Source: CAD feature listing. Evaluate the final solid. Frame: model axes, mm. Give positions to 0.01 mm unless a question says otherwise; leave off trailing zeros. Loops run counter-clockwise (first coordinate to the right, second up) from the corner with the lowest first, then second, coordinate; pieces in that order, holes last. Notation, with made-up numbers: M 72,60.5 L 113,60.5 A11 cw 113,68.5 Z; hole C 59,62 d7. An arc over 180 degrees is marked long. Answer in a Markdown table with one row per item.
```python
from build123d import *

# Parameters (mm, degrees)
F1_W     = 75
F1_H     = 75
F2_DEPTH = 0.45
F3_DEPTH = 0.451
F4_SCALE = 2
F5_R     = 10


with BuildPart() as f2:
    # F1 (on Top) → F2 (new body)
    with BuildSketch(Plane.XY):
        with Locations((42.972257086, 25.7581188657)):
            Rectangle(F1_W, F1_H)
    extrude(amount=F2_DEPTH)

    # F0 (on Top) → F3 (cut, through all)
    with BuildSketch(Plane.XY):
        with BuildLine():
            Line((20.8079852164, 34.7860567272), (63.291762352, 34.7860567272))
            ThreePointArc((63.291762352, 34.7860567272), (64.7059759144, 35.3718431648), (65.291762352, 36.7860567272))
            Line((65.291762352, 36.7860567272), (65.291762352, 39.0860567272))
            Line((65.291762352, 39.0860567272), (22.8079852164, 39.0860567272))
            ThreePointArc((22.8079852164, 39.0860567272), (21.393771654, 38.5002702895), (20.8079852164, 37.0860567272))
            Line((20.8079852164, 37.0860567272), (20.8079852164, 34.7860567272))
        make_face()
        with BuildLine():
            Line((38.5079852164, 14.3860567272), (38.5079852164, 32.2860567272))
            Line((38.5079852164, 32.2860567272), (31.5079852164, 32.2860567272))
            ThreePointArc((31.5079852164, 32.2860567272), (30.093771654, 31.7002702895), (29.5079852164, 30.2860567272))
            Line((29.5079852164, 30.2860567272), (29.5079852164, 12.3860567272))
            Line((29.5079852164, 12.3860567272), (36.5079852164, 12.3860567272))
            ThreePointArc((36.5079852164, 12.3860567272), (37.9221987788, 12.9718431648), (38.5079852164, 14.3860567272))
        make_face()
        with BuildLine():
            Line((54.1434029907, 27.9860567272), (54.1434029907, 32.2860567272))
            Line((54.1434029907, 32.2860567272), (47.1434029907, 32.2860567272))
            ThreePointArc((47.1434029907, 32.2860567272), (45.7291894283, 31.7002702895), (45.1434029907, 30.2860567272))
            Line((45.1434029907, 30.2860567272), (45.1434029907, 12.3860567272))
            Line((45.1434029907, 12.3860567272), (54.1434029907, 12.3860567272))
            Line((54.1434029907, 12.3860567272), (54.1434029907, 16.6860567272))
            Line((54.1434029907, 16.6860567272), (54.1434029907, 23.6860567272))
            Line((54.1434029907, 23.6860567272), (54.1434029907, 27.9860567272))
        make_face()
        with BuildLine():
            Line((65.291762352, 27.9860567272), (54.1434029907, 27.9860567272))
            Line((54.1434029907, 27.9860567272), (54.1434029907, 23.6860567272))
            Line((54.1434029907, 23.6860567272), (63.291762352, 23.6860567272))
            ThreePointArc((63.291762352, 23.6860567272), (64.7059759144, 24.2718431648), (65.291762352, 25.6860567272))
            Line((65.291762352, 25.6860567272), (65.291762352, 27.9860567272))
        make_face()
        with BuildLine():
            Line((65.291762352, 16.6860567272), (54.1434029907, 16.6860567272))
            Line((54.1434029907, 16.6860567272), (54.1434029907, 12.3860567272))
            Line((54.1434029907, 12.3860567272), (63.291762352, 12.3860567272))
            ThreePointArc((63.291762352, 12.3860567272), (64.7059759144, 12.9718431648), (65.291762352, 14.3860567272))
            Line((65.291762352, 14.3860567272), (65.291762352, 16.6860567272))
        make_face()
    extrude(amount=F3_DEPTH, mode=Mode.SUBTRACT)


with BuildPart() as f2_1:
    # F4: moved
    add(f2.part.scale(F4_SCALE))

    # F5
    f5_edges = [f2_1.edges().sort_by_distance(p)[0] for p in [
        (160.944514, -23.483762, 0.45),
        (10.944514, -23.483762, 0.45),
        (10.944514, 126.516238, 0.45),
        (160.944514, 126.516238, 0.45),
    ]]
    fillet(f5_edges, radius=F5_R)


solid = f2_1.part
```
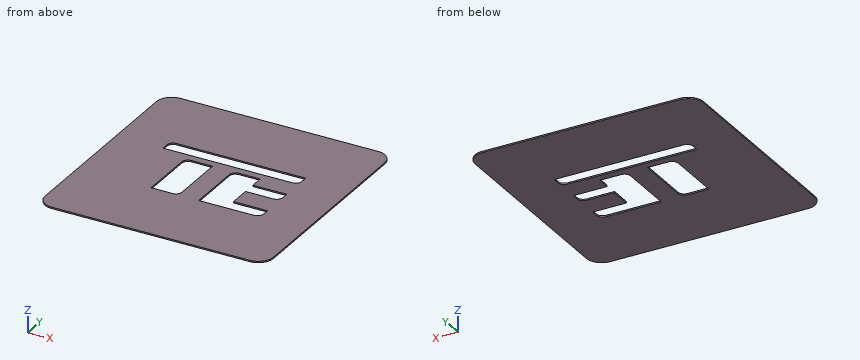
Q1. Section query C-C (y = 42.5). Output: boundary loops of the cut face in (x, z), plus the area to 3 significant figures.
Values follow:
| item | result |
|---|---|
| outline | M 10.94,0 L 59.02,0 L 59.02,0.9 L 10.94,0.9 Z; M 77.02,0 L 90.29,0 L 90.29,0.9 L 77.02,0.9 Z; M 108.29,0 L 160.94,0 L 160.94,0.9 L 108.29,0.9 Z |
| area | 103 mm^2 |
Q2. Section query B-B (z = 0.3). Give the number of separate pieces and of enclosed holes in the cut face, plus the area to 3 significant figures.
Values follow:
| item | result |
|---|---|
| separate pieces | 1 |
| enclosed holes | 3 |
| area | 19,900 mm^2 |
Q3. Ray query, probe 1 along X at (y, z) = (61, 0.65); probe 2 along Y at (x, z) = (118, 0.55); probe 3 along Y at (x, z) = (69.5, 0.8). Return the intervals inside material, ascending. Write a range as from..to.
Values follow:
| item | result |
|---|---|
| probe 1 | 10.94..59.04, 77.02..90.31, 108.29..160.94 |
| probe 2 | -23.48..24.77, 33.37..47.37, 55.97..69.57, 78.17..126.52 |
| probe 3 | -23.48..24.77, 64.57..69.57, 78.17..126.52 |
Q4. Section query A-A (x = 96). Output: boundary loops of the cut face in (y, z).
Values follow:
| item | result |
|---|---|
| outline | M -23.48,0 L 24.77,0 L 24.77,0.9 L -23.48,0.9 Z; M 64.57,0 L 69.57,0 L 69.57,0.9 L 64.57,0.9 Z; M 78.17,0 L 126.52,0 L 126.52,0.9 L 78.17,0.9 Z |
